Could you check a few things on this model? Use its own coordinates, in mm. Coordinates: 2 decimals unless noted, no trailing zeros. Write each loop counter-clockwise with the first axis right and the second up, starting at its lowest first coordinate (ties: lowest second). Pieces come first, ordered by that corner, then holes. Notation, with made-up numbers: (-23.5, -16.75) - (0.5, -16.75) arc R21 ccw to (0.5, 12.25) - close; hole circle Ø8 at (45.5, -32). An arc over 180 degrees is marked (long way). Answer as a JSON object with one key per item and string values. Group by question number.
1) Will these pins go through, and if not, where does the flat tip stop? pin 1 Ø8 at (y, z) = (-7, 7.5) entering from +X; pin 2 Ø1.5 at (y, z) = (-11, -6.5) entering from -X; pin 3 Ø1.5 at (x, y) = (-4, -5.5) entering from -Z; pin 4 Ø8 at (x, z) = (7.5, 5.5) entering from -Y.
2) We'd pull the mould along Y, two halves only. Please class faces 1 (the cylindrical face through (-7.084, -14.235, -1.573)), 2 (the cylindrical face through (8.406, -19.514, 5.36)), 3 (the flat face through (0, -25.07, 0)), 4 (the flat face through (0, 0, 0)): released by +Y, released by -Y, zero draft, split by the parting line, or undercut.
3) If we section it at B-B (x = 0): Write out the boundary of the cut face in (y, z), plus the area to 3 significant figures.
4) Please list where these lines run through material, in increasing order: line 1 along X through (y, z) = (-1.25, -2); line 2 along Z through (x, y) = (-8.5, -16.5); line 3 along Y through (x, z) = (-6.75, -5.75).
5) If we section it at C-C (y = -13): Write out the boundary of the cut face in (x, z).
6) If we section it at D-D (y = -18): Write out the boundary of the cut face in (x, z).
7) If we section it at A-A (z = 0): Write out the boundary of the cut face in (x, y), plus the area to 3 significant figures.
```python
from build123d import *

# Parameters (mm, degrees)
F2_SIZE = 1.524
F3_SIZE = 1.524
F4_R    = 0.381


with BuildPart() as f1:
    # F0 (on Right) → F1 (revolve)
    with BuildSketch(Plane.YZ):
        Polygon((-25.0698, 0), (0, 0), (0, 7.51078), (-13.462, 7.51078), (-13.462, 7.25678), (-14.986, 7.25678), (-14.986, 7.51078), (-14.986, 9.9695), (-25.0698, 9.9695), align=None)
    revolve(axis=Axis((0, -12.5349, 0), (0, 1, 0)))

    # F2
    f2_edges = [f1.edges().sort_by_distance(p)[0] for p in [
        (0, -25.0698, -9.9695),
    ]]
    chamfer(f2_edges, length=F2_SIZE)

    # F3
    f3_edges = [f1.edges().sort_by_distance(p)[0] for p in [
        (0, 0, -7.51078),
    ]]
    chamfer(f3_edges, length=F3_SIZE)

    # F4
    f4_edges = [f1.edges().sort_by_distance(p)[0] for p in [
        (0, -14.986, -9.9695),
    ]]
    fillet(f4_edges, radius=F4_R)


solid = f1.part
```
Here are the results:
{
 "1": {"pin 1": "stops at x = 6.65", "pin 2": "stops at x = -4.83", "pin 3": "stops at z = -6.77", "pin 4": "stops at y = -25.07"},
 "2": {"face 1": "undercut", "face 2": "zero draft", "face 3": "released by -Y", "face 4": "released by +Y"},
 "3": {"outline": "(-25.07, -8.45) - (-23.55, -9.97) - (-15.37, -9.97) arc R0.38 ccw to (-14.99, -9.59) - (-14.99, -7.26) - (-13.46, -7.26) - (-13.46, -7.51) - (-1.52, -7.51) - (0, -5.99) - (0, 5.99) - (-1.52, 7.51) - (-13.46, 7.51) - (-13.46, 7.26) - (-14.99, 7.26) - (-14.99, 9.59) arc R0.38 ccw to (-15.37, 9.97) - (-23.55, 9.97) - (-25.07, 8.45) - close", "area": "421 mm²"},
 "4": {"line 1": "x = -6.95 to 6.95", "line 2": "z = -5.21 to 5.21", "line 3": "y = -24.65 to -14.99"},
 "5": {"outline": "circle Ø15.02 at (0, 0)"},
 "6": {"outline": "circle Ø19.94 at (0, 0)"},
 "7": {"outline": "(-9.97, -23.55) - (-8.45, -25.07) - (8.45, -25.07) - (9.97, -23.55) - (9.97, -15.37) arc R0.38 ccw to (9.59, -14.99) - (7.26, -14.99) - (7.26, -13.46) - (7.51, -13.46) - (7.51, -1.52) - (5.99, 0) - (-5.99, 0) - (-7.51, -1.52) - (-7.51, -13.46) - (-7.26, -13.46) - (-7.26, -14.99) - (-9.59, -14.99) arc R0.38 ccw to (-9.97, -15.37) - close", "area": "421 mm²"}
}
